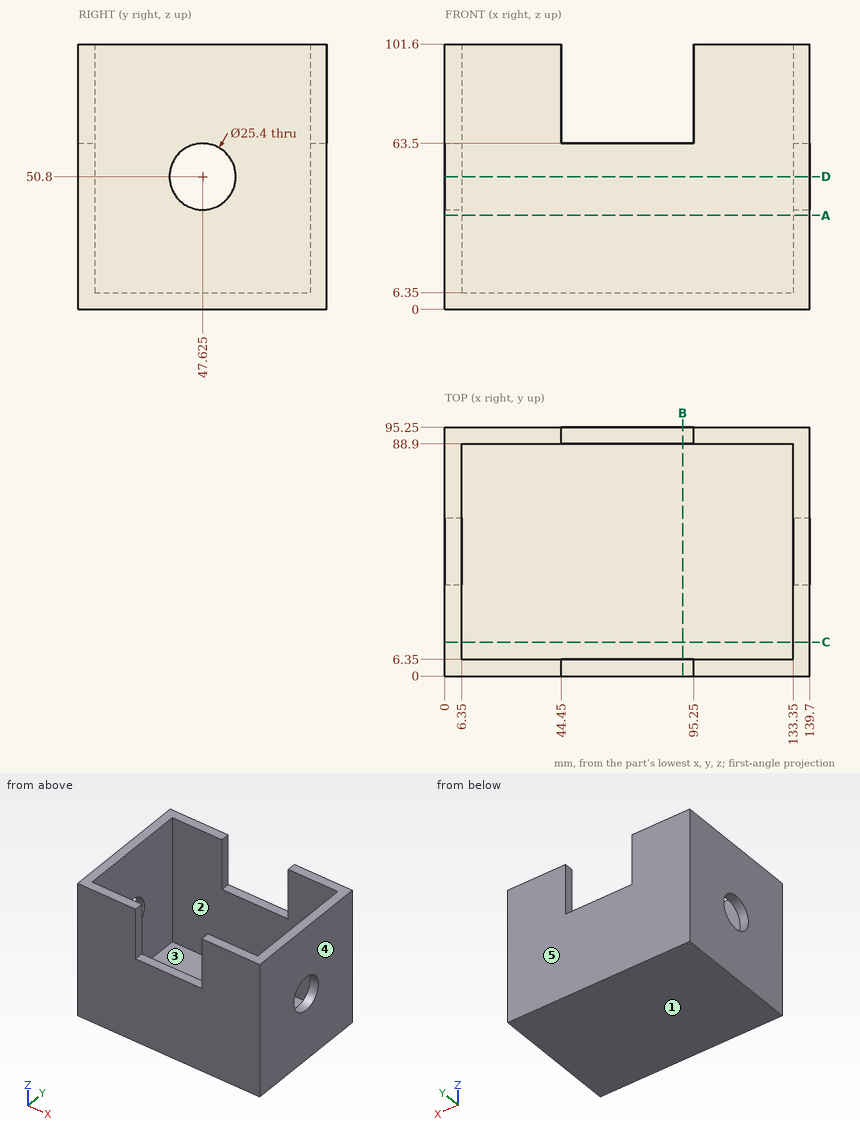
Geometry: see drawing. Coordinates: mm, zero at the bounding-box minimum. A direction names the side the tool comes from. Coordinates: 2 decimals unless noted, no trailing zeros. Loops run counter-clockwise (first coordinate to the right, second up) from the corner with the lowest first, then second, coordinate; pieces in that order, holes last.
(1) Section A-A on z = 36. Return the cut outline in (x, y), then the cut area to 3 significant figures.
(2) Material intervals for probe 1 along X at (y, z) = (28, 60); probe 2 along Y at (x, z) = (3, 50), sorted ascending.
(3) Pull-direction query (X, two-part tool) for the marked faces 3, 4 and 5; classes: released by +X, released by -X, zero draft, split by the parting line, or undercut.
(4) Section B-B on x = 91. Return the cut outline in (y, z).
(5) Section C-C on y = 13. Return the cut outline in (x, z).
(6) Set-up query: the marked faces 1 and 2. Return all of +Z, -Z, +X, -X, +Y, -Y with unobstructed straight access to the full face (end or side cutting, diameter ignored); none if empty.
(7) First-contact query: pin 1 Ø3 at (x, y) = (57.5, 92.5) entering from +Z; pin 2 Ø25 at (x, y) = (48, 57) entering from +Z. Flat tips, straight axial feed; report the tip coordinate or a pass-through.
(8) Section D-D on z = 50.8. Return the cut outline in (x, y) (3 decimals), then the cut area to 3 significant figures.
Data:
1. outline: (0, 0) - (139.7, 0) - (139.7, 95.25) - (0, 95.25) - close; hole (6.35, 6.35) - (133.35, 6.35) - (133.35, 88.9) - (6.35, 88.9) - close
1. area: 2,820 mm2
2. probe 1: x = 0 to 6.35, 133.35 to 139.7
2. probe 2: y = 0 to 34.95, 60.3 to 95.25
3. face 3: undercut
3. face 4: released by +X
3. face 5: zero draft
4. outline: (0, 0) - (95.25, 0) - (95.25, 63.5) - (88.9, 63.5) - (88.9, 6.35) - (6.35, 6.35) - (6.35, 63.5) - (0, 63.5) - close
5. outline: (0, 0) - (139.7, 0) - (139.7, 101.6) - (133.35, 101.6) - (133.35, 6.35) - (6.35, 6.35) - (6.35, 101.6) - (0, 101.6) - close
6. face 1: -Z, +X, -X, +Y, -Y
6. face 2: +Z
7. pin 1: stops at z = 63.5
7. pin 2: stops at z = 6.35
8. outline: (0, 0) - (139.7, 0) - (139.7, 34.925) - (133.35, 34.925) - (133.35, 6.35) - (6.35, 6.35) - (6.35, 34.925) - (0, 34.925) - close; (0, 60.325) - (6.35, 60.325) - (6.35, 88.9) - (133.35, 88.9) - (133.35, 60.325) - (139.7, 60.325) - (139.7, 95.25) - (0, 95.25) - close
8. area: 2,500 mm2
